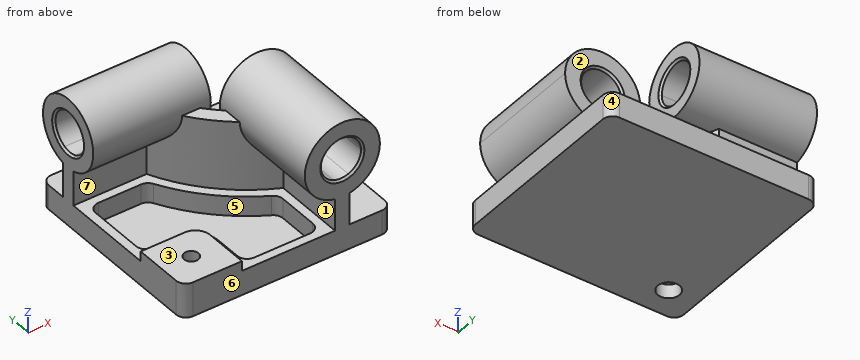
from build123d import *

# Parameters (mm, degrees)
F1_DEPTH       = 35
F2_DEPTH       = 25
F3_DEPTH       = 5
F4_DEPTH       = 95
F5_D           = 14.75
F5_CBORE_D     = 22.25
F5_CBORE_DEPTH = 14
F6_DEPTH       = 25
F8_DEPTH       = 120
F9_DEPTH       = 120
F11_DEPTH      = 120
F12_DEPTH      = 120
F13_SIZE       = 2


with BuildPart() as f1:
    # F0 (on Top) → F1 (new body)
    with BuildSketch(Plane.XY):
        with BuildLine():
            ThreePointArc((-106.5, 10), (-103.5710678119, 2.9289321881), (-96.5, 0))
            Line((-96.5, 0), (-46.5, 0))
            Line((-46.5, 0), (-46.5, 45))
            ThreePointArc((-46.5, 45), (-50.8933982822, 55.6066017178), (-61.5, 60))
            Line((-61.5, 60), (-106.5, 60))
            Line((-106.5, 60), (-106.5, 10))
        make_face()
    extrude(amount=F1_DEPTH)

    # F0 (on Top) → F2 (join)
    with BuildSketch(Plane.XY):
        with BuildLine():
            Line((-46.5, 45), (-46.5, 0))
            Line((-46.5, 0), (48.5, 0))
            Line((48.5, 0), (48.5, 9))
            Line((48.5, 9), (48.5, 73.0645805597))
            ThreePointArc((48.5, 73.0645805597), (0.9989947663, 106.8341893096), (-31.8154327598, 155))
            Line((-31.8154327598, 155), (-106.5, 155))
            Line((-106.5, 155), (-106.5, 60))
            Line((-106.5, 60), (-61.5, 60))
            ThreePointArc((-61.5, 60), (-50.8933982822, 55.6066017178), (-46.5, 45))
        make_face()
        with BuildLine():
            Line((-61.5, 69), (-87.5, 69))
            ThreePointArc((-87.5, 69), (-94.5710678119, 71.9289321881), (-97.5, 79))
            Line((-97.5, 79), (-97.5, 136))
            ThreePointArc((-97.5, 136), (-94.5710678119, 143.0710678119), (-87.5, 146))
            Line((-87.5, 146), (-44.0372922197, 146))
            ThreePointArc((-44.0372922197, 146), (-38.8802046252, 144.5676395548), (-35.2004786871, 140.6808895084))
            ThreePointArc((-35.2004786871, 140.6808895084), (-5.5795172138, 100.1842682312), (34.3477319863, 69.8001858066))
            ThreePointArc((34.3477319863, 69.8001858066), (38.1161859272, 66.1293498865), (39.5, 61.0537868568))
            Line((39.5, 61.0537868568), (39.5, 19))
            ThreePointArc((39.5, 19), (36.5710678119, 11.9289321881), (29.5, 9))
            Line((29.5, 9), (-27.5, 9))
            ThreePointArc((-27.5, 9), (-34.5710678119, 11.9289321881), (-37.5, 19))
            Line((-37.5, 19), (-37.5, 45))
            ThreePointArc((-37.5, 45), (-44.5294372515, 61.9705627485), (-61.5, 69))
        make_face(mode=Mode.SUBTRACT)
    extrude(amount=F2_DEPTH)

    # F0 (on Top) → F3 (join)
    with BuildSketch(Plane.XY):
        with BuildLine():
            ThreePointArc((-97.5, 79), (-94.5710678119, 71.9289321881), (-87.5, 69))
            Line((-87.5, 69), (-61.5, 69))
            ThreePointArc((-61.5, 69), (-44.5294372515, 61.9705627485), (-37.5, 45))
            Line((-37.5, 45), (-37.5, 19))
            ThreePointArc((-37.5, 19), (-34.5710678119, 11.9289321881), (-27.5, 9))
            Line((-27.5, 9), (29.5, 9))
            ThreePointArc((29.5, 9), (36.5710678119, 11.9289321881), (39.5, 19))
            Line((39.5, 19), (39.5, 61.0537868568))
            ThreePointArc((39.5, 61.0537868568), (38.1161859272, 66.1293498865), (34.3477319863, 69.8001858066))
            ThreePointArc((34.3477319863, 69.8001858066), (-5.5795172138, 100.1842682312), (-35.2004786871, 140.6808895084))
            ThreePointArc((-35.2004786871, 140.6808895084), (-38.8802046252, 144.5676395548), (-44.0372922197, 146))
            Line((-44.0372922197, 146), (-87.5, 146))
            ThreePointArc((-87.5, 146), (-94.5710678119, 143.0710678119), (-97.5, 136))
            Line((-97.5, 136), (-97.5, 79))
        make_face()
    extrude(amount=F3_DEPTH)

    # F0 (on Top) → F4 (join)
    with BuildSketch(Plane.XY):
        with BuildLine():
            Line((48.5, 9), (48.5, 0))
            Line((48.5, 0), (63.5, 0))
            Line((63.5, 0), (63.5, 80))
            ThreePointArc((63.5, 80), (11.2368967619, 117.7368967619), (-26.5, 170))
            Line((-26.5, 170), (-106.5, 170))
            Line((-106.5, 170), (-106.5, 155))
            Line((-106.5, 155), (-31.8154327598, 155))
            ThreePointArc((-31.8154327598, 155), (0.9989947663, 106.8341893096), (48.5, 73.0645805597))
            Line((48.5, 73.0645805597), (48.5, 9))
        make_face()
    extrude(amount=F4_DEPTH)

    # F5 (through all)
    with Locations(Plane(origin=(0, 0, 0), x_dir=(1, 0, 0), z_dir=(0, 0, -1))):
        with Locations((-76.5, -30)):
            CounterBoreHole(F5_D / 2, F5_CBORE_D / 2, F5_CBORE_DEPTH)

    # F0 (on Top) → F6 (join)
    with BuildSketch(Plane.XY):
        with BuildLine():
            Line((63.5, 80), (63.5, 0))
            Line((63.5, 0), (96.5, 0))
            ThreePointArc((96.5, 0), (103.5710678119, 2.9289321881), (106.5, 10))
            Line((106.5, 10), (106.5, 190))
            ThreePointArc((106.5, 190), (103.5710678119, 197.0710678119), (96.5, 200))
            Line((96.5, 200), (-96.5, 200))
            ThreePointArc((-96.5, 200), (-103.5710678119, 197.0710678119), (-106.5, 190))
            Line((-106.5, 190), (-106.5, 170))
            Line((-106.5, 170), (-26.5, 170))
            ThreePointArc((-26.5, 170), (11.2368967619, 117.7368967619), (63.5, 80))
        make_face()
    extrude(amount=F6_DEPTH)

    # F7 (on face) → F8 (cut)
    with BuildSketch(Plane.XZ):
        with BuildLine():
            Line((48.5, 75.9212159717), (48.5, 95))
            Line((48.5, 95), (63.5, 95))
            Line((63.5, 95), (63.5, 75.9212159717))
            ThreePointArc((63.5, 75.9212159717), (72.9410743461, 83.4566036194), (76.5, 95))
            ThreePointArc((76.5, 95), (44.4566036194, 111.9410743461), (48.5, 75.9212159717))
        make_face()
        with BuildLine():
            Line((63.5, 95), (48.5, 95))
            Line((48.5, 95), (48.5, 75.9212159717))
            ThreePointArc((48.5, 75.9212159717), (56, 74.5), (63.5, 75.9212159717))
            Line((63.5, 75.9212159717), (63.5, 95))
        make_face()
    extrude(amount=-F8_DEPTH, mode=Mode.SUBTRACT)

    # F7 (on face) → F9 (join)
    with BuildSketch(Plane.XZ):
        with BuildLine():
            Line((48.5, 57.4075197384), (48.5, 75.9212159717))
            ThreePointArc((48.5, 75.9212159717), (44.4566036194, 111.9410743461), (76.5, 95))
            ThreePointArc((76.5, 95), (72.9410743461, 83.4566036194), (63.5, 75.9212159717))
            Line((63.5, 75.9212159717), (63.5, 57.4075197384))
            ThreePointArc((63.5, 57.4075197384), (85.6390332562, 70.6900785715), (94.333335, 95))
            ThreePointArc((94.333335, 95), (31.6900785715, 124.6390332562), (48.5, 57.4075197384))
        make_face()
        with BuildLine():
            ThreePointArc((63.5, 75.9212159717), (56, 74.5), (48.5, 75.9212159717))
            Line((48.5, 75.9212159717), (48.5, 57.4075197384))
            ThreePointArc((48.5, 57.4075197384), (56, 56.666665), (63.5, 57.4075197384))
            Line((63.5, 57.4075197384), (63.5, 75.9212159717))
        make_face()
    extrude(amount=-F9_DEPTH)

    # F10 (on face) → F11 (cut)
    with BuildSketch(Plane(origin=(-106.5, 0, 0), x_dir=(0, -1, 0), z_dir=(-1, 0, 0))):
        with BuildLine():
            Line((-170, 95), (-155, 95))
            Line((-155, 95), (-155, 75.9212159717))
            ThreePointArc((-155, 75.9212159717), (-145.5589256539, 83.4566036194), (-142, 95))
            ThreePointArc((-142, 95), (-174.0433963806, 111.9410743461), (-170, 75.9212159717))
            Line((-170, 75.9212159717), (-170, 95))
        make_face()
        with BuildLine():
            Line((-155, 75.9212159717), (-155, 95))
            Line((-155, 95), (-170, 95))
            Line((-170, 95), (-170, 75.9212159717))
            ThreePointArc((-170, 75.9212159717), (-162.5, 74.5), (-155, 75.9212159717))
        make_face()
    extrude(amount=-F11_DEPTH, mode=Mode.SUBTRACT)

    # F10 (on face) → F12 (join)
    with BuildSketch(Plane(origin=(-106.5, 0, 0), x_dir=(0, -1, 0), z_dir=(-1, 0, 0))):
        with BuildLine():
            ThreePointArc((-142, 95), (-145.5589256539, 83.4566036194), (-155, 75.9212159717))
            Line((-155, 75.9212159717), (-155, 60.3012968542))
            ThreePointArc((-155, 60.3012968542), (-134.8730204329, 72.7065031904), (-127, 95))
            ThreePointArc((-127, 95), (-184.7934968096, 122.6269795671), (-170, 60.3012968542))
            Line((-170, 60.3012968542), (-170, 75.9212159717))
            ThreePointArc((-170, 75.9212159717), (-174.0433963806, 111.9410743461), (-142, 95))
        make_face()
        with BuildLine():
            Line((-155, 60.3012968542), (-155, 75.9212159717))
            ThreePointArc((-155, 75.9212159717), (-162.5, 74.5), (-170, 75.9212159717))
            Line((-170, 75.9212159717), (-170, 60.3012968542))
            ThreePointArc((-170, 60.3012968542), (-162.5, 59.5), (-155, 60.3012968542))
        make_face()
    extrude(amount=-F12_DEPTH)

    # F13
    f13_edges = [f1.edges().sort_by_distance(p)[0] for p in [
        (35.5, 0, 95),
        (35.5, 120, 95),
        (13.5, 183, 95),
        (-106.5, 162.5, 74.5),
        (-106.5, 145.558926, 83.456604),
        (-106.5, 174.043396, 111.941074),
    ]]
    chamfer(f13_edges, length=F13_SIZE)


solid = f1.part
The listing builds one solid part. Answer for the finished solid, in the listing's coordinates (mm). Face numbers are marked on the shaded views. A direction names the side the tool comes from. Round coordinates to 2 decimals unless told otherwise and drop trailing zeros. Loops run counter-clockwise (first coordinate to the right, second up) from the corner with the lowest first, then second, coordinate; pieces in that order, holes last. Notation, with made-up numbers: M 69,-17.5 L 88,-17.5 A25 ccw 88,0.5 Z; hole C 39,43.25 d5. An arc over 180 degrees is marked long. Return JSON: item names as keys, results as strings.
Q1. Find section D-D, the plane x = -91.5. Determine the outline of the cut face in (y, z), plus the area to 3 significant figures.
Results list:
{"outline": "M 0,0 L 200,0 L 200,25 L 170,25 L 170,60.3 A35.5 ccw long 155,60.3 L 155,25 L 145.17,25 L 145.17,5 L 69.83,5 L 69.83,25 L 60,25 L 60,35 L 0,35 Z; hole C 162.5,95 d41", "area": "7,250 mm2"}
Q2. Each of these flat-tipped pins is pushed along its axis until it touches: pin 1 Ø3 at (x, y) = (-57.5, 84) entering from +Z; pin 2 Ø4 at (x, z) = (-84, 60.5) entering from +Y; pin 3 Ø6.5 at (x, y) = (-81.5, 34) entering from -Z. Where does it stop, or does it pass through?
Results list:
{"pin 1": "stops at z = 5", "pin 2": "stops at y = 176.78", "pin 3": "stops at z = 14"}
Q3. Which of the six approach directions +Z, -Z, +X, -X, +Y, -Y give full straight-line access (tool end or side, diameter ignored) to the marked faces 1, 2 and 3?
Results list:
{"face 1": "-Y", "face 2": "+Z, +X, +Y", "face 3": "+Z, -X, -Y"}
Q4. Find section B-B, the plane x = 56. Determine the outline of the cut face in (y, z).
Results list:
{"outline": "M 0,0 L 200,0 L 200,25 L 83.97,25 L 83.97,56.67 L 120,56.67 L 120,72.5 L 118,74.5 L 2,74.5 L 0,72.5 Z; M 0,117.5 L 2,115.5 L 118,115.5 L 120,117.5 L 120,133.33 L 0,133.33 Z"}
Q5. Find the intervals of material crossed by line 1 along Y through (x, z) = (-76.5, 30.5) (3 decimals); line 2 along Z through (x, y) = (-69.5, 162.5); line 3 along Y through (x, z) = (-76, 9), in increasing order. Write a range as from..to.
Results list:
{"line 1": "y = 0..22.625, 37.375..60, 155..170", "line 2": "z = 0..74.5, 115.5..130.5", "line 3": "y = 0..18.89, 41.11..69, 146..200"}
Q6. The mould has two halves that part along Y. Classify the marked faces 4, 5, 6 and 7: released by +Y, released by -Y, zero draft, split by the parting line, or undercut.
Results list:
{"face 4": "released by +Y", "face 5": "undercut", "face 6": "released by -Y", "face 7": "undercut"}
Q7. Find section C-C, the plane z = 42.5. Determine the outline of the cut face in (x, y), plus the area to 3 significant figures.
Results list:
{"outline": "M -106.5,155 L -31.82,155 A165.17 ccw 48.5,73.06 L 48.5,0 L 63.5,0 L 63.5,80 A202.28 cw -26.5,170 L -106.5,170 Z", "area": "4,030 mm2"}
Q8. Find section A-A, the plane y = 30. Determine the outline of the cut face in (x, z) (3 decimals), plus the area to 3 significant figures.
Results list:
{"outline": "M -106.5,0 L -87.625,0 L -87.625,14 L -83.875,14 L -83.875,35 L -106.5,35 Z; M -69.125,14 L -65.375,14 L -65.375,0 L 106.5,0 L 106.5,25 L 63.5,25 L 63.5,57.408 A38.333 ccw long 48.5,57.408 L 48.5,25 L 39.5,25 L 39.5,5 L -37.5,5 L -37.5,25 L -46.5,25 L -46.5,35 L -69.125,35 Z; hole C 56,95 d41", "area": "7,540 mm2"}
